```python
from build123d import *

# Parameters (mm, degrees)
F0_W     = 203.487146
F0_H     = 135
F0_W_2   = 67
F0_H_2   = 38
F0_W_3   = 73
F0_H_3   = 58
F1_DEPTH = 3


with BuildPart() as f1:
    # F0 (on Top) → F1 (new body)
    with BuildSketch(Plane.XY):
        Polygon((-136, -19), (-87.5, -67.5), (-87.5, 67.5), (-136, 19), align=None)
        with Locations((14.243573, 0)):
            Rectangle(F0_W, F0_H)
        with Locations((-169.5, 0)):
            Rectangle(F0_W_2, F0_H_2)
        Polygon((115.987146, 67.5), (115.987146, -67.5), (130, -29), (130, 29), align=None)
        with Locations((166.5, 0)):
            Rectangle(F0_W_3, F0_H_3)
    extrude(amount=F1_DEPTH)


solid = f1.part
```
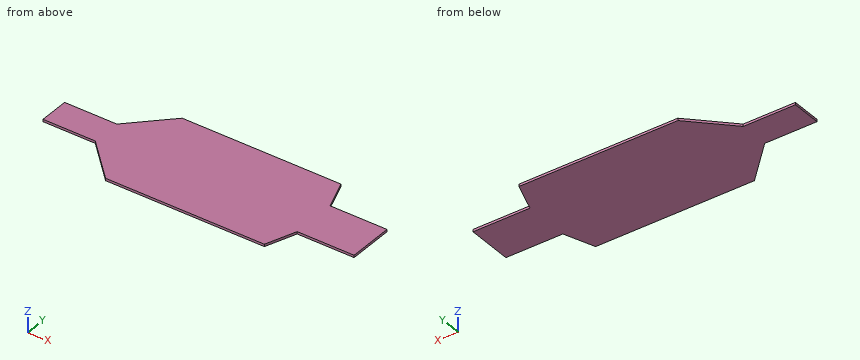
Part model, mm, in its own coordinate system. Round coordinates to 2 decimals unless told otherwise and drop trailing zeros. Write each loop counter-clockwise with the first axis right and the second up, starting at its lowest first coordinate (ties: lowest second). Pieces come first, ordered by that corner, then holes.
Item 1: Cut at A-A, the plane z = 0.5. Give the cut face in (x, y).
Results:
outline: (-203, -19) - (-136, -19) - (-87.5, -67.5) - (115.99, -67.5) - (130, -29) - (203, -29) - (203, 29) - (130, 29) - (115.99, 67.5) - (-87.5, 67.5) - (-136, 19) - (-203, 19) - close
Item 2: Drop flat-ended pins along their axis: pin 1 Ø1.5 at (x, z) = (-169.5, 1.5) entering from -Y; pin 2 Ø1.5 at (x, z) = (153, 2) entering from +Y. Give the stop position or say it passes through.
Results:
pin 1: stops at y = -19
pin 2: stops at y = 29
Item 3: Cut at C-C, the plane y = -42.5. Give the cut face in (x, z), plus the area to 3 significant figures.
Results:
outline: (-112.5, 0) - (125.09, 0) - (125.09, 3) - (-112.5, 3) - close
area: 713 mm2
Item 4: Probe L1, parallel to Y at x = -171, z = 2.15; L2, parallel to Y at x = 137.5, z = 1.3; L3, parallel to X at y = 40, z = 1.4. List the from-to ranges inside material, lowest first.
Results:
L1: y = -19 to 19
L2: y = -29 to 29
L3: x = -115 to 126
Item 5: Cut at B-B, the plane x = -128. Give the cut face in (y, z).
Results:
outline: (-27, 0) - (27, 0) - (27, 3) - (-27, 3) - close
